Source: CAD feature listing. Evaluate the final solid. Frame: model axes, mm. A direction names the side the tool comes from. Round coordinates to 2 decimals unless told otherwise and drop trailing zeros. Order: outer loops, then holes, each group sorted by start corner. A loop starts at its lowest first (then second) coordinate and runs counter-clockwise, first axis right, second up. Notation, with made-up numbers: M -30,-14.75 L -24,-14.75 A17 ccw -24,11.25 Z; hole C -8,80 d8. An arc over 180 degrees is marked long. Answer as CSV lines item,"result". Start each with the question number.
Item 1: Section query D-D on x = -5.25. Return the cut outline in (y, z).
Item 2: Section query A-A on z = 15.25. Return the cut outline in (x, y).
Item 3: Pull-direction query (Y, two-part tool) for faces 1 (the face through (-17, -6, 2.4)), 2 (the face through (-24, 6, 18)), 3 (the face through (-12, 3.4, 11)); classes: +Y half, -Y half, draft (parallel to the pull), parting line (faces both ways), or undercut.
Item 4: Set-up query: faces 4 (the face through (-12, 9, 11)), 5 (the face through (-1.91, -3.6, 3.21)), 6 (the face through (-12.18, 1.72, 9.9)), 7 (the face through (-14, 0, 9)). Return all of +Z, -Z, +X, -X, +Y, -Y with unobstructed straight access to the full face (end or side cutting, diameter ignored); none if empty.
Item 5: Section query B-B on y = -6. Return the cut outline in (x, z).
Item 6: Line query: line 1 (Y direction, x = -5.25, z = 2); line 2 (Y direction, x = -2.5, z = 11); line 3 (Y direction, x = -23.5, z = 7.75). Output: solid intervals per line, ascending. Write a range as [from, to].
Item 7: First-contact query: P1, Ø7.5, axis at x = -4.5, y = -4, coming from the +Z side; P2, Ø2.5, axis at x = -9.5, z = 13.5, coming from the -Y side; P3, Ø3, axis at x = -5.25, y = -4.65, coming from the +Z side; P4, Ø4, axis at x = -16, z = 10, coming from the -Y side. Flat tips, straight axial feed; report the tip coordinate or a pass-through.
Item 8: Section query C-C on z = 4.5. Return the cut outline in (x, y), plus the area to 3 significant figures.
from build123d import *

# Parameters (mm, degrees)
SKETCH1_W           = 24
SKETCH1_H           = 12.7
SKETCH1_R           = 1.5
BOSS_EXTRUDE1_DEPTH = 18
SKETCH3_R           = 6
CUT_EXTRUDE1_DEPTH  = 15
SKETCH4_R           = 8.1
CUT_EXTRUDE2_DEPTH  = 3.7
CUT_EXTRUDE3_START  = -3.4
SKETCH5_R           = 8.1
CUT_EXTRUDE3_DEPTH  = 3.4
SKETCH6_W           = 24
SKETCH6_H           = 4
BOSS_EXTRUDE2_DEPTH = 8.6
SKETCH7_R           = 2
CUT_EXTRUDE4_DEPTH  = 8.6
SKETCH8_R           = 3.5
CUT_EXTRUDE5_DEPTH  = 1.6
BOSS_EXTRUDE3_DEPTH = 3.5


with BuildPart() as part:
    # Sketch1 → Boss-Extrude1 (new body)
    with BuildSketch(Plane.XY):
        with Locations((-12, 6.35)):
            Rectangle(SKETCH1_W, SKETCH1_H)
        with Locations((-21.5, 6.05)):
            Circle(SKETCH1_R, mode=Mode.SUBTRACT)
        with Locations((-2.5, 6.35)):
            Circle(SKETCH1_R, mode=Mode.SUBTRACT)
    extrude(amount=BOSS_EXTRUDE1_DEPTH)

    # Sketch3 → Cut-Extrude1 (cut)
    with BuildSketch(Plane(origin=(0, 12.7, 0), x_dir=(1, 0, 0), z_dir=(0, 1, 0))):
        with Locations((-12, -18)):
            Circle(SKETCH3_R)
    extrude(amount=-CUT_EXTRUDE1_DEPTH, mode=Mode.SUBTRACT)

    # Sketch4 → Cut-Extrude2 (cut)
    with BuildSketch(Plane(origin=(0, 12.7, 0), x_dir=(1, 0, 0), z_dir=(0, 1, 0))):
        with Locations((-12, -18)):
            Circle(SKETCH4_R)
    extrude(amount=-CUT_EXTRUDE2_DEPTH, mode=Mode.SUBTRACT)

    # Sketch5 → Cut-Extrude3 (cut)
    with BuildSketch(Plane.XZ.offset(CUT_EXTRUDE3_START)):
        with Locations((-12, 18)):
            Circle(SKETCH5_R)
    extrude(amount=CUT_EXTRUDE3_DEPTH, mode=Mode.SUBTRACT)

    # Sketch6 → Boss-Extrude2 (add)
    with BuildSketch(Plane.XZ):
        with Locations((-12, 2)):
            Rectangle(SKETCH6_W, SKETCH6_H)
    extrude(amount=BOSS_EXTRUDE2_DEPTH)

    # Sketch7 → Cut-Extrude4 (cut)
    with BuildSketch(Plane.XY.offset(4)):
        with Locations((-18.75, -4.65)):
            Circle(SKETCH7_R)
        with Locations((-5.25, -4.65)):
            Circle(SKETCH7_R)
    extrude(amount=-CUT_EXTRUDE4_DEPTH, mode=Mode.SUBTRACT)

    # Sketch8 → Cut-Extrude5 (cut)
    with BuildSketch(Plane.XY.offset(4)):
        with Locations((-18.75, -4.65)):
            Circle(SKETCH8_R)
        with Locations((-5.25, -4.65)):
            Circle(SKETCH8_R)
    extrude(amount=-CUT_EXTRUDE5_DEPTH, mode=Mode.SUBTRACT)

    # Sketch9 → Boss-Extrude3 (add)
    with BuildSketch(Plane.ZY.offset(24)):
        Polygon((0, 12.7), (0, -8.6), (4, -8.6), (4, 0), (18, 0), (18, 12.7), align=None)
    extrude(amount=BOSS_EXTRUDE3_DEPTH)


solid = part.part
Results:
1,outline,"M -8.6,0 L -6.65,0 L -6.65,2.4 L -8.15,2.4 L -8.15,4 L -8.6,4 Z; M -2.65,0 L 12.7,0 L 12.7,13.52 L 9,13.52 L 9,18 L 3.4,18 L 3.4,13.52 L 0,13.52 L 0,4 L -1.15,4 L -1.15,2.4 L -2.65,2.4 Z"
2,outline,"M -27.5,0 L -19.62,0 L -19.62,3.4 L -17.33,3.4 L -17.33,9 L -19.62,9 L -19.62,12.7 L -27.5,12.7 Z; M -6.67,3.4 L -4.38,3.4 L -4.38,0 L 0,0 L 0,12.7 L -4.38,12.7 L -4.38,9 L -6.67,9 Z; hole C -21.5,6.05 d3; hole C -2.5,6.35 d3"
3,face 1,"undercut"
3,face 2,"draft"
3,face 3,"-Y half"
4,face 4,"+Z, +Y"
4,face 5,"+Z"
4,face 6,"+Z, -Y"
4,face 7,"+Z, +X, -X, -Y"
5,outline,"M -27.5,0 L -20.23,0 L -20.23,2.4 L -21.98,2.4 L -21.98,4 L -27.5,4 Z; M -17.27,0 L -6.73,0 L -6.73,2.4 L -8.48,2.4 L -8.48,4 L -15.52,4 L -15.52,2.4 L -17.27,2.4 Z; M -3.77,0 L 0,0 L 0,4 L -2.02,4 L -2.02,2.4 L -3.77,2.4 Z"
6,line 1,"[-8.6, -6.65], [-2.65, 12.7]"
6,line 2,"[0, 4.85], [7.85, 12.7]"
6,line 3,"[0, 12.7]"
7,P1,"z = 4"
7,P2,"y = 3.4"
7,P3,"through"
7,P4,"y = 0"
8,outline,"M -27.5,0 L 0,0 L 0,12.7 L -27.5,12.7 Z; hole C -21.5,6.05 d3; hole C -2.5,6.35 d3"
8,area,"335 mm^2"
